Check sheet for the modelled part. Datum: model origin and axes. Units: mm. A direction names the side the tool comes from. Coordinates: 2 decimals unless noted, no trailing zeros. Write each loop counter-clockwise with the first axis right and the second up, starting at its lowest first coordinate (ties: lowest second). Pieces come first, ordered by that corner, then holes. Notation, with made-up numbers: (64, 87.25) - (118, 87.25) arc R5 ccw to (118, 96.25) - close; hole circle Ø7 at (32, 60.5). An arc over 180 degrees is marked (long way). Use one line per item in the form item = value. Start each with the question number.
1. Cross-section at D-D on x = 2.75. Give the number of separate pieces and of enclosed holes in the cut face, then the cut area to 3 significant figures.
2. Cross-section at A-A on y = 10.5. Record the boundary of the cut face in (x, z) (3 decimals).
3. Cross-section at B-B on y = 2.5. Record the boundary of the cut face in (x, z) (1 decimal).
4. Go/stop test with flat-tipped pins: pin 1 Ø1.5 at (x, y) = (8, 17) entering from -Z; pin 2 Ø2.5 at (x, z) = (4.76, -3.18) entering from -Y; pin 3 Ø0.6 at (y, z) = (6.7, -10.52) entering from -X; pin 4 Ø3 at (x, y) = (3, 11) entering from +Z. Record where each tip stops, or that it passes through.
5. Scan lines: line 1 along Z through (x, y) = (9, 12.5); line 2 along Z through (x, y) = (4.5, 14.75); line 3 along Y through (x, z) = (8, -3). Record each from-to range of solid material in increasing order.
6. Draft check along Z on faces 5 (the face through (5, 0, -42)), 6 (the face through (5, 2, 0)), 7 (the face through (4.177, 2.415, -3.712)), 8 (the face through (5, 12, -42.428)). Enter one of: +Z half, -Z half, draft (parallel to the pull), parting line (faces both ways), or undercut.
7. Tool access check on faces 1 (the face through (3.13, 6.38, -38.73)), 2 (the face through (6, 4.762, -3)), 3 (the face through (4.7, 4.762, -46.4)), 4 (the face through (5, 7, -12.785)). Record the directions out of +Z, -Z, +X, -X, +Y, -Y that give a thin tool (end or side, any length) a straight path to the whole face; none if there is none.
```python
from build123d import *

# Parameters (mm, degrees)
BOSS_EXTRUDE1_DEPTH = 9.525
CUT_EXTRUDE1_REACH  = 6.763
SKETCH2_R           = 0.508
SKETCH2_R_2         = 0.79375
SKETCH3_R           = 0.508
CUT_EXTRUDE2_DEPTH  = 6.35
FILLET1_R           = 1.5875


with BuildPart() as part:
    # Sketch1 → Boss-Extrude1 (new body)
    with BuildSketch(Plane(origin=(0, 0, 0), x_dir=(0, 0, -1), z_dir=(1, 0, 0))):
        Polygon((0, 0), (12.7847852, 0), (12.7847852, 13.390245), (36.0778552, 13.390245), (36.0778552, 0), (48.8626404, 0), (48.8626404, 4.7625), (42.4278552, 4.7625), (42.4278552, 19.740245), (41.4309052, 19.740245), (6.3509652, 19.740245), (6.3509652, 4.7625), (0, 4.7625), align=None)
    extrude(amount=BOSS_EXTRUDE1_DEPTH)

    # Sketch2 → Cut-Extrude1 (cut, up to next)
    with BuildSketch(Plane(origin=(0, 4.7625, 0), x_dir=(1, 0, 0), z_dir=(0, 1, 0)), mode=Mode.PRIVATE) as cut_extrude1_sk1:
        with Locations((4.7625, 45.6876404)):
            Circle(SKETCH2_R)
    cut_extrude1_tool1 = extrude(cut_extrude1_sk1.sketch, amount=-CUT_EXTRUDE1_REACH, mode=Mode.PRIVATE) & part.part
    add(cut_extrude1_tool1.solids().sort_by_distance((4.7625, 4.7625, -45.68764))[0], mode=Mode.SUBTRACT)
    # Sketch2 → Cut-Extrude1 (cut, up to next)
    with BuildSketch(Plane(origin=(0, 4.7625, 0), x_dir=(1, 0, 0), z_dir=(0, 1, 0)), mode=Mode.PRIVATE) as cut_extrude1_sk2:
        with Locations((4.7625, 3.1756604)):
            Circle(SKETCH2_R_2)
    cut_extrude1_tool2 = extrude(cut_extrude1_sk2.sketch, amount=-CUT_EXTRUDE1_REACH, mode=Mode.PRIVATE) & part.part
    add(cut_extrude1_tool2.solids().sort_by_distance((4.7625, 4.7625, -3.17566))[0], mode=Mode.SUBTRACT)

    # Sketch3 → Cut-Extrude2 (cut)
    with BuildSketch(Plane.ZY):
        with Locations((-38.3232152, 6.68528)):
            Circle(SKETCH3_R)
        with Locations((-10.5229152, 6.6951225)):
            Circle(SKETCH3_R)
    extrude(amount=-CUT_EXTRUDE2_DEPTH, mode=Mode.SUBTRACT)

    # Fillet1
    fillet1_edges = [part.edges().sort_by_distance(p)[0] for p in [
        (4.7625, 4.7625, 0),
        (4.7625, 4.7625, -6.3509652),
        (4.7625, 19.740245, -6.3509652),
        (4.7625, 19.740245, -42.4278552),
        (4.7625, 4.7625, -42.4278552),
        (4.7625, 4.7625, -48.8626404),
    ]]
    fillet(fillet1_edges, radius=FILLET1_R)


solid = part.part
```
Final values:
q1.separate_pieces = 1
q1.enclosed_holes = 2
q1.area = 458 mm²
q2.outline = (0, -42.428) - (9.525, -42.428) - (9.525, -36.078) - (0, -36.078) - close; (0, -12.785) - (9.525, -12.785) - (9.525, -6.351) - (0, -6.351) - close
q3.outline = (0, -48.9) - (9.5, -48.9) - (9.5, -36.1) - (0, -36.1) - close; (0, -12.8) - (9.5, -12.8) - (9.5, 0) - (0, 0) - close; hole circle Ø1.6 at (4.8, -3.2); hole circle Ø1 at (4.8, -45.7)
q4.pin_1 = -42.43
q4.pin_2 = 0
q4.pin_3 = 6.35
q4.pin_4 = -6.35
q5.line_1 = -42.43 to -36.08, -12.78 to -6.35
q5.line_2 = -42.43 to -6.35
q5.line_3 = 0 to 4.76
q6.face_5 = draft
q6.face_6 = +Z half
q6.face_7 = undercut
q6.face_8 = -Z half
q7.face_1 = -X
q7.face_2 = +Z, +X, -X, +Y
q7.face_3 = -Z, +X, -X, +Y
q7.face_4 = +X, -X, -Y
